Autodesk Inventor part; units mm, degrees
ref_plane "YZ Plane" through (0, 0, 0) normal (1, 0, 0) x (0, 1, 0)
ref_plane "XZ Plane" through (0, 0, 0) normal (0, 1, 0) x (-1, 0, 0)
ref_plane "XY Plane" through (0, 0, 0) normal (0, 0, 1) x (1, 0, 0)
sketch "Skizze1" plane through (0, 0, 0) normal (0, 1, 0) x (-1, 0, 0)
  line L0 (0, 0) -> (0, -6)
  line L1 (0, -20) -> (0, -26)
  line L2 (0, -26) -> (2, -26)
  line L3 (2, -26) -> (2, -20.746)
  line L4 (0, 0) -> (2, 0)
  line L5 (2, 0) -> (2, -5.254)
  arc A0 (3, -16) -> (3, -10) centre (3, -13) ccw
  line L6 (6, -13) -> (8, -13)
  line L7 (2, -26) -> (2, -19)
  arc A1 (3.5, -18.8095) -> (3.5, -7.1905) centre (2, -13) ccw
  arc A2 (3.5, -18.8095) -> (2, -20.746) centre (4, -20.746) ccw
  arc A3 (2, -5.254) -> (3.5, -7.1905) centre (4, -5.254) ccw
  line L8 (3, -16) -> (3, -16)
  line L9 (0, -19) -> (0, -20)
  line L10 (3, -10) -> (3, -10)
  line L11 (0, -7) -> (0, -6)
  arc A4 (3, -16) -> (0, -19) centre (3, -19) ccw
  arc A5 (0, -7) -> (3, -10) centre (3, -7) ccw
  point P0 (0, -10)
  point P1 (0, -16)
  point P2 (2, -19)
  point P3 (2, -7)
  dimension "d0" = 10
  dimension "d1" = 3
  dimension "d3" = 10
  dimension "d4" = 2
  dimension "d5" = 7
  dimension "d6" = 2
  dimension "d7" = 7
  dimension "d9" = 3
  dimension "d23" = 2
  dimension "d24" = 7
  dimension "d25" = 2
  dimension "d26" = 3
extrude "Extrusion1" add sketch "Skizze1" along normal blind 10
sketch "Skizze2" plane through (-2, 0, -5) normal (-1, 0, 0) x (0, 0, 1)
  line L0 (5, 0) -> (5, 10)
  line L1 (5, 5) -> (2.5, 5)
  line L2 (-21, 0) -> (-21, 10)
  line L3 (-21, 5) -> (-18.5, 5)
  dimension "d14" = 2.5
  dimension "d15" = 2.5
hole "Bohrung1" at (-2, 5, -2.5) at (-2, 5, -23.5) direction (1, 0, 0) diameter 3 depth 8 tip angle 118
properties part number "Draht_Halterung"
Check sheet for the modelled part. Datum: model origin and axes. Units: mm. A direction names the side the tool comes from. Round coordinates to 2 decimals unless told otherwise and drop trailing zeros. Order: outer loops, then holes, each group sorted by start corner. A loop starts at its lowest first (then second) coordinate and runs counter-clockwise, first axis right, second up. Notation, with made-up numbers: (40, 8.5) - (85, 8.5) arc R22 ccw to (85, 35.5) - close; hole circle Ø9 at (19, 53.25). An arc over 180 degrees is marked (long way). Write item = value, one per line.
Q1. Section check B-B (y = 5). Record the boundary of the cut face in (x, z).
Computed:
outline = (-3.5, -18.81) arc R2 cw to (-2, -20.75) - (-2, -22) - (0, -22) - (0, -19) arc R3 ccw to (-3, -16) arc R3 cw to (-3, -10) arc R3 ccw to (0, -7) - (0, -4) - (-2, -4) - (-2, -5.25) arc R2 cw to (-3.5, -7.19) arc R6 ccw to start; (-2, -26) - (0, -26) - (0, -25) - (-2, -25) - close; (-2, -1) - (0, -1) - (0, 0) - (-2, 0) - close
Q2. Draft check along Z on faces 1 (the face through (0, 4.9, -21.7)), 2 (the face through (-1, 5, -1)), 3 (the face through (-8, 5, -13)). Enter one of: pulls with the +Z half, pulls with the -Z half, needs draft (parallel to the pull), parting line crosses it, or undercut.
Computed:
face_1 = needs draft
face_2 = undercut
face_3 = parting line crosses it
Q3. Section check C-C (y = 0.75). Record the boundary of the cut face in (x, z), and give its area (3 significant figures).
Computed:
outline = (-3.5, -18.81) arc R2 cw to (-2, -20.75) - (-2, -26) - (0, -26) - (0, -19) arc R3 ccw to (-3, -16) arc R3 cw to (-3, -10) arc R3 ccw to (0, -7) - (0, 0) - (-2, 0) - (-2, -5.25) arc R2 cw to (-3.5, -7.19) arc R6 ccw to start
area = 73.7 mm^2
Q4. Tool access check on faces 4 (the face through (-2, 4, -4)), 5 (the face through (-5.5, 10, -11)), 6 (the face through (-2, 4, -22)). Record the directions out of +Z, -Z, +X, -X, +Y, -Y that give a thin tool (end or side, any length) a straight path to the whole face; none if there is none.
Computed:
face_4 = +Z, -X, +Y, -Y
face_5 = +Z, -Z, +X, -X, +Y
face_6 = -Z, -X, +Y, -Y
Q5. Section check D-D (x = -4.25). Record the boundary of the cut face in (y, z).
Computed:
outline = (0, -18.56) - (10, -18.56) - (10, -15.73) - (0, -15.73) - close; (0, -10.27) - (10, -10.27) - (10, -7.44) - (0, -7.44) - close
Q6. Go/stop test with flat-tipped pins: pin 1 (4 mm diameter, centred on x = -3, y = 1, fed in from -Z); pin 2 (1.8 mm diameter, centred on y = 5, z = -2.5, fed in from -X); pin 3 (2.5 mm diameter, centred on y = 7.5, z = -2, fed in from -X); pin 4 (6 mm diameter, centred on y = 4.5, z = -11, fed in from +X). Record where each tip stops, or that it passes through.
Computed:
pin_1 = -26
pin_2 = through
pin_3 = -2
pin_4 = -0.17
Q7. Thickness scan on line 1 along Z through (x, y) = (-1.15, 5); line 2 along Y through (x, z) = (-0.5, -2.5); line 3 along Z through (x, y) = (-1, 5). Record the ranges inside material, lowest first.
Computed:
line_1 = -26 to -25, -22 to -16.64, -9.36 to -4, -1 to 0
line_2 = 0 to 3.5, 6.5 to 10
line_3 = -26 to -25, -22 to -16.76, -9.24 to -4, -1 to 0
Q8. Section check A-A (z = -2.5). Record the boundary of the cut face in (x, y).
Computed:
outline = (-2, 0) - (0, 0) - (0, 3.5) - (-2, 3.5) - close; (-2, 6.5) - (0, 6.5) - (0, 10) - (-2, 10) - close
